```python
from build123d import *

# Parameters (mm, degrees)
SKETCH1_W           = 60
SKETCH1_H           = 60
BOSS_EXTRUDE1_DEPTH = 5
SKETCH3_R           = 29.5
BOSS_EXTRUDE2_DEPTH = 21
SKETCH4_R           = 25
BOSS_EXTRUDE3_DEPTH = 7
SKETCH5_R           = 22.5
BOSS_EXTRUDE4_DEPTH = 62
CUT_EXTRUDE1_REACH  = 106.043
SKETCH6_R           = 2
SKETCH7_R           = 12
BOSS_EXTRUDE5_DEPTH = 6
BOSS_EXTRUDE6_START = -6
SKETCH8_R           = 4
BOSS_EXTRUDE6_DEPTH = 30
SKETCH9_R           = 2.5
SKETCH9_W           = 2
SKETCH9_H           = 5
BOSS_EXTRUDE7_DEPTH = 10


with BuildPart() as part:
    # Sketch1 → Boss-Extrude1 (new body)
    with BuildSketch(Plane(origin=(0, 0, 0), x_dir=(0, 0, -1), z_dir=(1, 0, 0))):
        Rectangle(SKETCH1_W, SKETCH1_H)
    extrude(amount=BOSS_EXTRUDE1_DEPTH)

    # Sketch3 → Boss-Extrude2 (add)
    with BuildSketch(Plane.ZY):
        with Locations(Location((0, 0, 0), (0, 0, 180))):
            Circle(SKETCH3_R)
    extrude(amount=BOSS_EXTRUDE2_DEPTH)

    # Sketch4 → Boss-Extrude3 (add)
    with BuildSketch(Plane.ZY.offset(21)):
        Circle(SKETCH4_R)
    extrude(amount=BOSS_EXTRUDE3_DEPTH)

    # Sketch5 → Boss-Extrude4 (add)
    with BuildSketch(Plane.ZY.offset(28)):
        Circle(SKETCH5_R)
    extrude(amount=BOSS_EXTRUDE4_DEPTH)

    # Sketch6 → Cut-Extrude1 (cut, up to next)
    with BuildSketch(Plane(origin=(5, 0, 0), x_dir=(0, 0, -1), z_dir=(1, 0, 0)), mode=Mode.PRIVATE) as cut_extrude1_sk1:
        with Locations((-25, 25)):
            Circle(SKETCH6_R)
    cut_extrude1_tool1 = extrude(cut_extrude1_sk1.sketch, amount=-CUT_EXTRUDE1_REACH, mode=Mode.PRIVATE) & part.part
    # Sketch6 → Cut-Extrude1 (cut, up to next)
    with BuildSketch(Plane(origin=(5, 0, 0), x_dir=(0, 0, -1), z_dir=(1, 0, 0)), mode=Mode.PRIVATE) as cut_extrude1_sk2:
        with Locations((25, 25)):
            Circle(SKETCH6_R)
    cut_extrude1_tool2 = extrude(cut_extrude1_sk2.sketch, amount=-CUT_EXTRUDE1_REACH, mode=Mode.PRIVATE) & part.part
    # Sketch6 → Cut-Extrude1 (cut, up to next)
    with BuildSketch(Plane(origin=(5, 0, 0), x_dir=(0, 0, -1), z_dir=(1, 0, 0)), mode=Mode.PRIVATE) as cut_extrude1_sk3:
        with Locations((25, -25)):
            Circle(SKETCH6_R)
    cut_extrude1_tool3 = extrude(cut_extrude1_sk3.sketch, amount=-CUT_EXTRUDE1_REACH, mode=Mode.PRIVATE) & part.part
    # Sketch6 → Cut-Extrude1 (cut, up to next)
    with BuildSketch(Plane(origin=(5, 0, 0), x_dir=(0, 0, -1), z_dir=(1, 0, 0)), mode=Mode.PRIVATE) as cut_extrude1_sk4:
        with Locations((-25, -25)):
            Circle(SKETCH6_R)
    cut_extrude1_tool4 = extrude(cut_extrude1_sk4.sketch, amount=-CUT_EXTRUDE1_REACH, mode=Mode.PRIVATE) & part.part
    add(cut_extrude1_tool1.solids().sort_by_distance((5, 25, 25))[0], mode=Mode.SUBTRACT)
    add(cut_extrude1_tool2.solids().sort_by_distance((5, 25, -25))[0], mode=Mode.SUBTRACT)
    add(cut_extrude1_tool3.solids().sort_by_distance((5, -25, -25))[0], mode=Mode.SUBTRACT)
    add(cut_extrude1_tool4.solids().sort_by_distance((5, -25, 25))[0], mode=Mode.SUBTRACT)

    # Sketch7 → Boss-Extrude5 (add)
    with BuildSketch(Plane(origin=(5, 0, 0), x_dir=(0, 0, -1), z_dir=(1, 0, 0))):
        Circle(SKETCH7_R)
    extrude(amount=BOSS_EXTRUDE5_DEPTH)

    # Sketch8 → Boss-Extrude6 (add)
    with BuildSketch(Plane(origin=(11, 0, 0), x_dir=(0, 0, -1), z_dir=(1, 0, 0)).offset(BOSS_EXTRUDE6_START)):
        Circle(SKETCH8_R)
    extrude(amount=BOSS_EXTRUDE6_DEPTH)

    # Sketch9 → Boss-Extrude7 (add)
    with BuildSketch(Plane.ZY.offset(90)):
        Circle(SKETCH9_R)
        with Locations((-16, 0)):
            Rectangle(SKETCH9_W, SKETCH9_H)
        with Locations((16, 0)):
            Rectangle(SKETCH9_W, SKETCH9_H)
    extrude(amount=BOSS_EXTRUDE7_DEPTH)


solid = part.part
```
Geometry check sheet. Reference: the model listing, model coordinates, mm. A direction names the side the tool comes from. Coordinates: 2 decimals unless noted, no trailing zeros. Order: outer loops, then holes, each group sorted by start corner. A loop starts at its lowest first (then second) coordinate and runs counter-clockwise, first axis right, second up.
Q1. Sectioned sample at B-B on x = -45. Record the cut outline in (y, z), and give its area (3 significant figures).
Reply:
outline: circle Ø45 at (0, 0)
area: 1,590 mm2
Q2. Sectioned sample at C-C on z = -18.5. Record the cut outline in (x, y), and give its area (3 significant figures).
Reply:
outline: (-90, -12.81) - (-28, -12.81) - (-28, -16.82) - (-21, -16.82) - (-21, -22.98) - (0, -22.98) - (0, -30) - (5, -30) - (5, 30) - (0, 30) - (0, 22.98) - (-21, 22.98) - (-21, 16.82) - (-28, 16.82) - (-28, 12.81) - (-90, 12.81) - close
area: 3,090 mm2
Q3. Thickness scan on probe 1 along Y at (x, z) = (2.5, -25); probe 2 along X at (y, z) = (27, -2); probe 3 along X at (y, z) = (2, 11). Record the ranges inside material, lowest first.
Reply:
probe 1: y = -30 to -27, -23 to 23, 27 to 30
probe 2: x = -21 to 5
probe 3: x = -90 to 11
Q4. Tool access check on faces 1 (the face through (-95, 0, -17)), 2 (the face through (-95, 0, 17)), 3 (the face through (5, 0, 14)), 4 (the face through (-28, 3.82, -22.34)). Record the directions out of +Z, -Z, +X, -X, +Y, -Y that give a thin tool (end or side, any length) a straight path to the whole face; none if there is none.
Reply:
face 1: -Z, -X, +Y, -Y
face 2: +Z, -X, +Y, -Y
face 3: +X
face 4: -X
Q5. Sectioned sample at A-A on z = 0. Record the cut outline in (x, y), and give its area (4 significant figures).
Reply:
outline: (-100, -2.5) - (-90, -2.5) - (-90, -22.5) - (-28, -22.5) - (-28, -25) - (-21, -25) - (-21, -29.5) - (0, -29.5) - (0, -30) - (5, -30) - (5, -12) - (11, -12) - (11, -4) - (35, -4) - (35, 4) - (11, 4) - (11, 12) - (5, 12) - (5, 30) - (0, 30) - (0, 29.5) - (-21, 29.5) - (-21, 25) - (-28, 25) - (-28, 22.5) - (-90, 22.5) - (-90, 2.5) - (-100, 2.5) - close
area: 5,065 mm2
Q6. Draft check along Z on faces 5 (the face through (-21, -13, 22)), 6 (the face through (2, 0, 30)), 7 (the face through (-95, 0, 15)), 8 (the face through (22.832, -3.905, 0.867)). Enter one of: released by +Z, released by -Z, zero draft, split by the parting line, or undercut.
Reply:
face 5: zero draft
face 6: released by +Z
face 7: undercut
face 8: split by the parting line
Q7. Depth check by flat-ended pin: pin 1 Ø0.6 at (x, z) = (-97, -16) entering from -Y; pin 2 Ø5 at (x, z) = (19.5, -0.5) entering from -Y; pin 3 Ø3.5 at (y, z) = (-25, 25) entering from +X; pin 4 Ø1.5 at (x, y) = (-97, 0.5) entering from +Z. Enter the tip coordinate at first touch or a pass-through.
Reply:
pin 1: stops at y = -2.5
pin 2: stops at y = -4
pin 3: passes through
pin 4: stops at z = 17
